The model under review builds one solid part; all positions refer to its coordinate system, in mm. A direction names the side the tool comes from. Give positions to 0.01 mm unless a question says otherwise; leave off trailing zeros. Order: outer loops, then holes, each group sorted by start corner. A loop starts at its lowest first (then second) coordinate and runs counter-clockwise, first axis right, second up. Notation, with made-up numbers: M 16,0 L 63,0 A12 cw 63,15 Z; hole C 65.25,66.5 d5. An arc over 180 degrees is marked long. One line per question, with ' | ' between items. Start each with the question number.
1. Insertion check: P1, Ø4, axis at x = -128, y = 39, coming from the -Z side. The pin has a flat end and moves straight along its axis. Give the tip position at first contact, or say it passes through.
2. We need section B-B on z = 12.25. Write out the cut boundary in (x, y), then the cut area to 3 significant figures.
3. We need section D-D on y = 103. Write out the cut boundary in (x, z), then the cut area to 3 significant figures.
4. We need section A-A on y = -50.8. Count the separate pieces of the cut face and the enclosed holes in it, then the cut area to 3 significant figures.
5. We need section C-C on y = 0. Write out the cut boundary in (x, z) (3 decimals).
6. The part is to be moulded in two halves that separate along Y. For faces 1 (the face through (3, 139.7, 13)), 2 (the face through (58.64, -79.2, 3.22)), 3 (the face through (199.38, -136.08, 12.88)), say which applies: +Y half, -Y half, draft (parallel to the pull), parting line (faces both ways), or undercut.
7. For faces 4 (the face through (-61.77, 86.14, 3.22)), 5 (the face through (-190.5, -2, 13)), list the 3-axis set-ups (+Z, -Z, +X, -X, +Y, -Y) from which the entire face can be reached by the end or side of a thin tool; tool diameter is ignored.
8. Wall thickness on L1, parallel to Z at x = -177, y = 101.5; L2, parallel to X at y = -5, z = 12.75; L3, parallel to X at y = -76.2, z = 3 (3 decimals): over which ranges is each line inside the solid? List them lowest first.
```python
from build123d import *

# Parameters (mm, degrees)
F1_DEPTH = 6.35
F2_DEPTH = 12.7
F4_D     = 8.89
F4_DEPTH = 12.7
F4_TIP   = 2.6708254516


# Not quite as in the source:
# - a feature names something its author has since deleted; it is built from what else it names


with BuildPart() as f1:
    # F0 (on Top) → F1 (new body)
    with BuildSketch(Plane.XY):
        with BuildLine():
            Line((190.5, 139.7), (0, 139.7))
            Line((0, 139.7), (-190.5, 139.7))
            ThreePointArc((-190.5, 139.7), (-199.4802561211, 135.9802561211), (-203.2, 127))
            Line((-203.2, 127), (-203.2, 0))
            Line((-203.2, 0), (-203.2, -127))
            ThreePointArc((-203.2, -127), (-199.4802561211, -135.9802561211), (-190.5, -139.7))
            Line((-190.5, -139.7), (0, -139.7))
            Line((0, -139.7), (190.5, -139.7))
            ThreePointArc((190.5, -139.7), (199.4802561211, -135.9802561211), (203.2, -127))
            Line((203.2, -127), (203.2, 0))
            Line((203.2, 0), (203.2, 127))
            ThreePointArc((203.2, 127), (199.4802561211, 135.9802561211), (190.5, 139.7))
        make_face()
        with BuildLine():
            ThreePointArc((177.8, 127), (186.7802561211, 123.2802561211), (190.5, 114.3))
            Line((190.5, 114.3), (190.5, -114.3))
            ThreePointArc((190.5, -114.3), (186.7802561211, -123.2802561211), (177.8, -127))
            Line((177.8, -127), (-177.8, -127))
            ThreePointArc((-177.8, -127), (-186.7802561211, -123.2802561211), (-190.5, -114.3))
            Line((-190.5, -114.3), (-190.5, 114.3))
            ThreePointArc((-190.5, 114.3), (-186.7802561211, 123.2802561211), (-177.8, 127))
            Line((-177.8, 127), (177.8, 127))
        make_face(mode=Mode.SUBTRACT)
        with BuildLine():
            Line((190.5, -114.3), (190.5, 114.3))
            ThreePointArc((190.5, 114.3), (186.7802561211, 123.2802561211), (177.8, 127))
            Line((177.8, 127), (-177.8, 127))
            ThreePointArc((-177.8, 127), (-186.7802561211, 123.2802561211), (-190.5, 114.3))
            Line((-190.5, 114.3), (-190.5, -114.3))
            ThreePointArc((-190.5, -114.3), (-186.7802561211, -123.2802561211), (-177.8, -127))
            Line((-177.8, -127), (177.8, -127))
            ThreePointArc((177.8, -127), (186.7802561211, -123.2802561211), (190.5, -114.3))
        make_face()
    extrude(amount=F1_DEPTH)

    # F0 (on Top) → F2 (join)
    with BuildSketch(Plane.XY):
        with BuildLine():
            Line((190.5, 139.7), (0, 139.7))
            Line((0, 139.7), (-190.5, 139.7))
            ThreePointArc((-190.5, 139.7), (-199.4802561211, 135.9802561211), (-203.2, 127))
            Line((-203.2, 127), (-203.2, 0))
            Line((-203.2, 0), (-203.2, -127))
            ThreePointArc((-203.2, -127), (-199.4802561211, -135.9802561211), (-190.5, -139.7))
            Line((-190.5, -139.7), (0, -139.7))
            Line((0, -139.7), (190.5, -139.7))
            ThreePointArc((190.5, -139.7), (199.4802561211, -135.9802561211), (203.2, -127))
            Line((203.2, -127), (203.2, 0))
            Line((203.2, 0), (203.2, 127))
            ThreePointArc((203.2, 127), (199.4802561211, 135.9802561211), (190.5, 139.7))
        make_face()
        with BuildLine():
            ThreePointArc((177.8, 127), (186.7802561211, 123.2802561211), (190.5, 114.3))
            Line((190.5, 114.3), (190.5, -114.3))
            ThreePointArc((190.5, -114.3), (186.7802561211, -123.2802561211), (177.8, -127))
            Line((177.8, -127), (-177.8, -127))
            ThreePointArc((-177.8, -127), (-186.7802561211, -123.2802561211), (-190.5, -114.3))
            Line((-190.5, -114.3), (-190.5, 114.3))
            ThreePointArc((-190.5, 114.3), (-186.7802561211, 123.2802561211), (-177.8, 127))
            Line((-177.8, 127), (177.8, 127))
        make_face(mode=Mode.SUBTRACT)
    extrude(amount=F2_DEPTH)

    # F4
    with Locations(Plane(origin=(0, 0, 0), x_dir=(1, 0, 0), z_dir=(0, 0, -1))):
        with Locations((18.4541802113, 25.4), (-18.4541802113, 25.4), (-29.8594908165, -9.7019366858), (0, -31.3961266285), (29.8594908165, -9.7019366858), (0, 0), (-36.9083604227, 50.8), (0, 50.8), (36.9083604227, 50.8), (59.7189816329, -19.4038733715), (0, -62.792253257), (-59.7189816329, -19.4038733715), (-72.4705065417, 23.5470949714), (-55.362540634, 76.2), (0, 76.2), (55.362540634, 76.2), (72.4705065417, 23.5470949714), (89.5784724494, -29.1058100573), (44.7892362247, -61.6470949714), (0, -94.1883798855), (-44.7892362247, -61.6470949714), (-89.5784724494, -29.1058100573), (-48.3136710278, 15.6980633142), (-29.8594908165, -41.0980633142), (29.8594908165, -41.0980633142), (48.3136710278, 15.6980633142), (-96.6273420556, 31.3961266285), (-119.4379632658, -38.807746743), (-59.7189816329, -82.1961266285), (59.7189816329, -82.1961266285), (119.4379632658, -38.807746743), (96.6273420556, 31.3961266285)):
            Hole(F4_D / 2, depth=F4_DEPTH)
            with Locations((0, 0, -(F4_DEPTH + F4_TIP / 2))):  # 118° drill point
                Cone(0, F4_D / 2, F4_TIP, mode=Mode.SUBTRACT)

    # F5: F1 across face


with BuildPart() as f1_1:
    add(f1.part)
    add(f1.part.mirror(Plane.XY.offset(12.7)))


solid = f1_1.part
```
Entries:
1) P1: stops at z = 0
2) outline: M -203.2,-127 A12.7 ccw -190.5,-139.7 L 190.5,-139.7 A12.7 ccw 203.2,-127 L 203.2,127 A12.7 ccw 190.5,139.7 L -190.5,139.7 A12.7 ccw -203.2,127 Z; hole M -190.5,-114.3 A12.7 ccw -177.8,-127 L 177.8,-127 A12.7 ccw 190.5,-114.3 L 190.5,114.3 A12.7 ccw 177.8,127 L -177.8,127 A12.7 ccw -190.5,114.3 Z | area: 16,800 mm^2
3) outline: M -203.2,0 L 203.2,0 L 203.2,25.4 L -203.2,25.4 Z; hole M -190.5,6.35 L 190.5,6.35 L 190.5,19.05 L -190.5,19.05 Z | area: 5,480 mm^2
4) separate pieces: 6 | enclosed holes: 0 | area: 5,150 mm^2
5) outline: M -203.2,0 L -4.445,0 L -4.445,6.35 L -190.5,6.35 L -190.5,19.05 L -4.445,19.05 L -4.445,25.4 L -203.2,25.4 Z; M 4.445,0 L 203.2,0 L 203.2,25.4 L 4.445,25.4 L 4.445,19.05 L 190.5,19.05 L 190.5,6.35 L 4.445,6.35 Z
6) face 1: +Y half | face 2: undercut | face 3: -Y half
7) face 4: +Z, -Z | face 5: none
8) L1: z = 0 to 6.35, 19.05 to 25.4 | L2: x = -203.2 to -190.5, 190.5 to 203.2 | L3: x = -203.2 to -59.808, -50.918 to -4.445, 4.445 to 50.918, 59.808 to 203.2
